```python
from build123d import *

# Parameters (mm, degrees)
ESQUISSE1_W             = 180
ESQUISSE1_H             = 110
BOSS_EXTRU_1_DEPTH      = 5
ESQUISSE2_W             = 20
ESQUISSE2_H             = 10
ESQUISSE2_W_2           = 5
ESQUISSE2_H_2           = 25
ENL_V_MAT_EXTRU_1_DEPTH = 5
ESQUISSE3_R             = 6
ENL_V_MAT_EXTRU_2_DEPTH = 5


with BuildPart() as part:
    # Esquisse1 → Boss.-Extru.1 (new body)
    with BuildSketch(Plane(origin=(0, 0, 0), x_dir=(1, 0, 0), z_dir=(0, 1, 0))):
        Rectangle(ESQUISSE1_W, ESQUISSE1_H)
    extrude(amount=BOSS_EXTRU_1_DEPTH)

    # Esquisse2 → Enlèv. mat.-Extru.1 (cut)
    with BuildSketch(Plane(origin=(0, 5, 0), x_dir=(1, 0, 0), z_dir=(0, 1, 0))):
        Polygon((-90, 55), (-90, 27.5), (-85, 27.5), (-85, 45), (-50, 45), (-50, 55), align=None)
        Polygon((85, 27.5), (90, 27.5), (90, 55), (50, 55), (50, 45), (85, 45), align=None)
        with Locations((20, 50)):
            Rectangle(ESQUISSE2_W, ESQUISSE2_H)
        with Locations((-20, 50)):
            Rectangle(ESQUISSE2_W, ESQUISSE2_H)
        with Locations((-87.5, 0)):
            Rectangle(ESQUISSE2_W_2, ESQUISSE2_H_2)
        Polygon((-90, -55), (-50, -55), (-50, -45), (-85, -45), (-85, -27.5), (-90, -27.5), align=None)
        Polygon((50, -45), (50, -55), (90, -55), (90, -27.5), (85, -27.5), (85, -45), align=None)
        with Locations((87.5, 0)):
            Rectangle(ESQUISSE2_W_2, ESQUISSE2_H_2)
        with Locations((20, -50)):
            Rectangle(ESQUISSE2_W, ESQUISSE2_H)
        with Locations((-20, -50)):
            Rectangle(ESQUISSE2_W, ESQUISSE2_H)
    extrude(amount=-ENL_V_MAT_EXTRU_1_DEPTH, mode=Mode.SUBTRACT)

    # Esquisse3 → Enlèv. mat.-Extru.2 (cut)
    with BuildSketch(Plane(origin=(0, 5, 0), x_dir=(1, 0, 0), z_dir=(0, 1, 0))):
        with Locations(Location((-35, 25, 0), (0, 0, 270))):
            Circle(ESQUISSE3_R)
        with Locations(Location((-35, 0, 0), (0, 0, 270))):
            Circle(ESQUISSE3_R)
        with Locations(Location((5, 25, 0), (0, 0, 270))):
            Circle(ESQUISSE3_R)
        with Locations(Location((5, 0, 0), (0, 0, 270))):
            Circle(ESQUISSE3_R)
        with Locations(Location((-65, 25, 0), (0, 0, 270))):
            Circle(ESQUISSE3_R)
        with Locations(Location((-65, 0, 0), (0, 0, 270))):
            Circle(ESQUISSE3_R)
    extrude(amount=-ENL_V_MAT_EXTRU_2_DEPTH, mode=Mode.SUBTRACT)


solid = part.part
```
Can you work these out from the model? Positions are in its coordinate system, mm. A direction names the side the tool comes from. Coordinates: 2 decimals unless noted, no trailing zeros. Loops run counter-clockwise (first coordinate to the right, second up) from the corner with the lowest first, then second, coordinate; pieces in that order, holes last.
1) Imagine slicing it at D-D on y = 1.3. State how many separate pieces and enclosed holes the cut face has, plus the area to 3 significant figures.
2) I need wall thicknesses on probe 1 along X at (y, z) = (3, -25); probe 2 along X at (y, z) = (1.9, 0.5); probe 3 along X at (y, z) = (1.1, 46). Which ranges of each line are inside material? Lowest first, please.
3) For pin 1 (2.5 mm diameter, centred on x = 74, y = 1.5, fed in from +Z); pin 2 (1.5 mm diameter, centred on y = 3, z = 51, fed in from +X); pin 3 (7 mm diameter, centred on x = -65, z = -25, fed in from -Y); pin 4 (2.5 mm diameter, centred on y = 2, z = 39.5, fed in from +X), each with a flat end and sliding along its axis, tell me the tip position at first contact or that it passes through.
4) Imagine slicing it at B-B on z = 0. List the corners of the cut face in (x, y) for me, plus the area to 3 significant figures.
5) Which directions (+Z, -Z, +X, -X, +Y, -Y) give clear straight access to the entire face, cutting with the end or side of a thin tool? Please do faces 1 (the flat face through (-68, 3, -45)), 2 (the flat face through (85, 3, 36)), 3 (the flat face through (-88, 3, -12.5)), 4 (the flat face through (-30, 3, 50)), 5 (the flat face through (10, 3, -50)).
6) Imagine slicing it at C-C on x = -35. List the corners of the cut face in (y, z) for me.
7) Imagine slicing it at A-A on x = -65. List the corners of the cut face in (y, z) for me, plus the area to 3 significant figures.
8) Thinking about a two-plate mould opening in Z: for faces 6 (the flat face through (50, 3, 50)), 7 (the flat face through (87, 3, -12.5)), 8 (the flat face through (-88, 3, -27.5)), 9 (the flat face through (20, 3, 45)), which applies, pulls with the +Z half, pulls with the -Z half, needs draft (parallel to the pull), parting line crosses it, or undercut?
Completed:
1. separate pieces: 1
1. enclosed holes: 6
1. area: 16,100 mm2
2. probe 1: x = -90 to -71, -59 to -41, -29 to -1, 11 to 90
2. probe 2: x = -85 to -70.98, -59.02 to -40.98, -29.02 to -0.98, 10.98 to 85
2. probe 3: x = -50 to -30, -10 to 10, 30 to 50
3. pin 1: stops at z = 45
3. pin 2: stops at x = 50
3. pin 3: passes through
3. pin 4: stops at x = 85
4. outline: (-85, 0) - (-71, 0) - (-71, 5) - (-85, 5) - close; (-59, 0) - (-41, 0) - (-41, 5) - (-59, 5) - close; (-29, 0) - (-1, 0) - (-1, 5) - (-29, 5) - close; (11, 0) - (85, 0) - (85, 5) - (11, 5) - close
4. area: 670 mm2
5. face 1: -Z, -X, +Y, -Y
5. face 2: +Z, +X, +Y, -Y
5. face 3: -X, +Y, -Y
5. face 4: +Z, +Y, -Y
5. face 5: -Z, +Y, -Y
6. outline: (0, -55) - (5, -55) - (5, -31) - (0, -31) - close; (0, -19) - (5, -19) - (5, -6) - (0, -6) - close; (0, 6) - (5, 6) - (5, 55) - (0, 55) - close
7. outline: (0, -45) - (5, -45) - (5, -31) - (0, -31) - close; (0, -19) - (5, -19) - (5, -6) - (0, -6) - close; (0, 6) - (5, 6) - (5, 45) - (0, 45) - close
7. area: 330 mm2
8. face 6: needs draft
8. face 7: undercut
8. face 8: pulls with the -Z half
8. face 9: pulls with the +Z half
